The listing builds one solid part. Answer for the finished solid, in the listing's coordinates (mm). A direction names the side the tool comes from. Give positions to 0.01 mm unless a question says otherwise; leave off trailing zeros. Loops run counter-clockwise (first coordinate to the right, second up) from the corner with the lowest first, then second, coordinate; pieces in that order, holes last.
Item 1: Section A-A, the plane x = 1.5 is taken. Give the vertices of the cut face in (y, z).
Item 2: Consider line 1 along X through (y, z) = (-2.25, 2.25); line 2 along Z through (x, y) = (6.25, -1.25); line 3 along Z through (x, y) = (0, 0.75). Determine where each line is inside the solid, lowest interval first.
Item 3: A tool of negligible diameter and unlimited length cuts with its end or side. For faces 1 (the face through (-7.44, 1.68, 2.9)), 2 (the face through (0.98, 0.53, -1.67)), from which of +Z, -Z, +X, -X, +Y, -Y can it reach the whole face along a straight path? Write none if from no direction.
from build123d import *

# Parameters (mm, degrees)
SKETCH5_R           = 1.7526
BOSS_EXTRUDE3_DEPTH = 12.7
CHAMFER1_SIZE       = 0.5953125
BOSS_EXTRUDE4_DEPTH = 2.38125
SKETCH8_OUTSIDE_W   = 67.644
SKETCH8_OUTSIDE_H   = 68.626
SKETCH8_OUTSIDE_R   = 3.175
CUT_EXTRUDE3_DEPTH  = 16.08125
CUT_EXTRUDE3_TAPER  = 60
CUT_EXTRUDE4_DEPTH  = 0.254
CIRPATTERN1_COUNT   = 6


with BuildPart() as part:
    # Sketch5 → Boss-Extrude3 (new body)
    with BuildSketch(Plane(origin=(7.540625, 0, 0), x_dir=(0, 0, -1), z_dir=(1, 0, 0))):
        Circle(SKETCH5_R)
    extrude(amount=-BOSS_EXTRUDE3_DEPTH)

    # Chamfer1
    chamfer1_edges = [part.edges().sort_by_distance(p)[0] for p in [
        (7.540625, 0, 1.7526),
    ]]
    chamfer(chamfer1_edges, length=CHAMFER1_SIZE)

    # Sketch6 → Boss-Extrude4 (add)
    with BuildSketch(Plane.ZY.offset(5.159375)):
        Polygon((3.175, 1.833087105), (0, 3.666174209), (-3.175, 1.833087105), (-3.175, -1.833087105), (0, -3.666174209), (3.175, -1.833087105), align=None)
    extrude(amount=BOSS_EXTRUDE4_DEPTH)

    # Sketch8 outside → Cut-Extrude3 (cut, through all)
    with BuildSketch(Plane.ZY.offset(7.540625)):
        Rectangle(SKETCH8_OUTSIDE_W, SKETCH8_OUTSIDE_H)
        Circle(SKETCH8_OUTSIDE_R, mode=Mode.SUBTRACT)
    extrude(amount=-CUT_EXTRUDE3_DEPTH, taper=CUT_EXTRUDE3_TAPER, mode=Mode.SUBTRACT)

    # Sketch12 → Cut-Extrude4 (cut)
    with BuildSketch(Plane.ZY.offset(7.540625)):
        with BuildLine():
            Line((0.09525, 2.44475), (0.09525, 1.36525))
            ThreePointArc((0.09525, 1.36525), (0, 1.27), (-0.09525, 1.36525))
            Line((-0.09525, 1.36525), (-0.09525, 2.44475))
            ThreePointArc((-0.09525, 2.44475), (0, 2.54), (0.09525, 2.44475))
        make_face()
    cut_extrude4 = extrude(amount=-CUT_EXTRUDE4_DEPTH, mode=Mode.SUBTRACT)

    # CirPattern1: Cut-Extrude4 ×6 about axis
    cirpattern1_axis = Axis((0, 0, 0), (1, 0, 0))
    for i in range(1, CIRPATTERN1_COUNT):
        add(cut_extrude4.rotate(cirpattern1_axis, i * 360 / CIRPATTERN1_COUNT), mode=Mode.SUBTRACT)


solid = part.part
Worked answers:
1. outline: circle Ø3.51 at (0, 0)
2. line 1: x = -7.54 to -5.16
2. line 2: z = -1.23 to 1.23
2. line 3: z = -1.58 to 1.58
3. face 1: +Z, -X, +Y
3. face 2: +X
